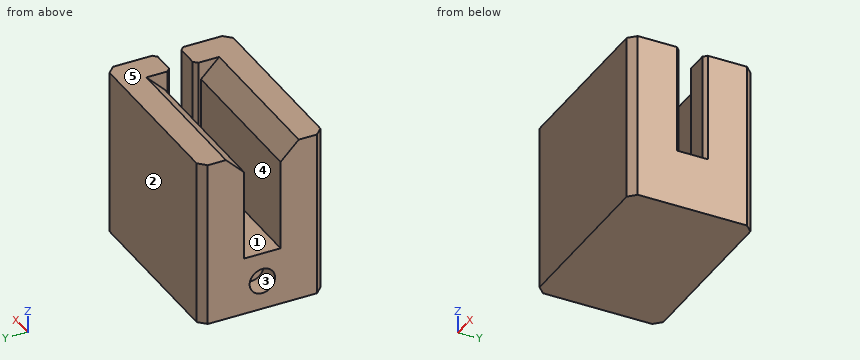
from build123d import *

# Parameters (mm, degrees)
F1_DEPTH = 34
F2_W     = 6.5
F2_H     = 30
F3_DEPTH = 8
F4_R     = 3.5
F5_DEPTH = 6
F6_W     = 42
F6_H     = 12
F7_DEPTH = 30
F8_SIZE  = 5
F9_SIZE  = 2
F10_SIZE = 1


with BuildPart() as f1:
    # F0 (on Front) → F1 (new body)
    with BuildSketch(Plane.XZ):
        Polygon((-20, 8), (-25, 8), (-25, -8), (25, -8), (25, 38), (17, 38), (17, 8), align=None)
    extrude(amount=F1_DEPTH)

    # F2 (on face) → F3 (cut, through all)
    with BuildSketch(Plane.YZ.offset(25)):
        with Locations((-17, 23)):
            Rectangle(F2_W, F2_H)
    extrude(amount=-F3_DEPTH, mode=Mode.SUBTRACT)

    # F4 (on face) → F5 (cut)
    with BuildSketch(Plane(origin=(-25, 0, 0), x_dir=(0, -1, 0), z_dir=(-1, 0, 0))):
        with Locations((17, 0)):
            Circle(F4_R)
    extrude(amount=-F5_DEPTH, mode=Mode.SUBTRACT)

    # F6 (on face) → F7 (join, through all)
    with BuildSketch(Plane.XY.offset(8)):
        with Locations((-4, -28)):
            Rectangle(F6_W, F6_H)
        with Locations((-4, -6)):
            Rectangle(F6_W, F6_H)
    extrude(amount=F7_DEPTH)

    # F8
    f8_edges = [f1.edges().sort_by_distance(p)[0] for p in [
        (-4, -22, 38),
        (-4, -12, 38),
    ]]
    chamfer(f8_edges, length=F8_SIZE)

    # F9
    f9_edges = [f1.edges().sort_by_distance(p)[0] for p in [
        (25, -34, 15),
        (25, 0, 15),
        (-25, -34, 15),
        (-25, 0, 15),
    ]]
    chamfer(f9_edges, length=F9_SIZE)

    # F10
    f10_edges = [f1.edges().sort_by_distance(p)[0] for p in [
        (17, -13.75, 23),
        (17, -20.25, 23),
        (25, -13.75, 23),
        (25, -20.25, 23),
    ]]
    chamfer(f10_edges, length=F10_SIZE)


solid = f1.part
Source: CAD feature listing. Evaluate the final solid. Frame: model axes, mm. Face numbers are marked on the shaded views. A direction names the side the tool comes from. Give positions to 0.01 mm unless a question says otherwise; leave off trailing zeros. Loops run counter-clockwise (first coordinate to the right, second up) from the corner with the lowest first, then second, coordinate; pieces in that order, holes last. Notation, with made-up numbers: (39, 12.5) -> (50, 12.5) arc R11 ccw to (50, 26.5) -> close; hole circle Ø8 at (75.25, -40). An arc over 180 degrees is marked (long way). Use a Markdown table: item, result. Add a question column.
1) Section query C-C, the plane z = 35. Return the cut outline in (x, y).
2) First-contact query: pin 1 (4 mm diameter, centred on x = -20, y = -11, fed in from +Z); pin 2 (1 mm diameter, centred on x = 16, y = -20, fed in from +Z); pin 3 (2 mm diameter, centred on y = -18, z = -1, fed in from -X); pin 4 (11 mm diameter, centred on y = -17, z = 0, fed in from -X). Flat tips, straight axial feed; report the tip coordinate or a pass-through.
3) Section query B-B, the plane x = -11. Return the cut outline in (y, z), then the cut area to 3 significant figures.
4) Section query D-D, the plane y = -17. Return the cut outline in (x, z).
5) Reachability of the marked faces 4 and 5 from +Z, -Z, +X, -X, +Y, -Y: full face, straight path, thin tool, end or side. Return the list, or none.
6) Section query A-A, the plane z = 27. Return the cut outline in (x, y).
7) Pull-direction query (Z, two-part tool) for the marked faces 1, 2 and 3; classes: +Z half, -Z half, draft (parallel to the pull), parting line (faces both ways), or undercut.
8) Line query: line 1 along Y through (x, z) = (14, 13.5); line 2 along Z through (x, y) = (-20.7, -17); line 3 along Z through (x, y) = (-11, -18). Output: solid intervals per line, ascending. Write a range as [from, to].
Numbers:
| question | item | result |
|---|---|---|
| 1 | outline | (-25, -32) -> (-23, -34) -> (23, -34) -> (25, -32) -> (25, -21.25) -> (24, -20.25) -> (18, -20.25) -> (17, -21.25) -> (17, -24) -> (-25, -24) -> close; (-25, -10) -> (17, -10) -> (17, -12.75) -> (18, -13.75) -> (24, -13.75) -> (25, -12.75) -> (25, -2) -> (23, 0) -> (-23, 0) -> (-25, -2) -> close |
| 2 | pin 1 | stops at z = 36 |
| 2 | pin 2 | stops at z = 8 |
| 2 | pin 3 | stops at x = -19 |
| 2 | pin 4 | stops at x = -25 |
| 3 | outline | (-34, -8) -> (0, -8) -> (0, 38) -> (-7, 38) -> (-12, 33) -> (-12, 8) -> (-22, 8) -> (-22, 33) -> (-27, 38) -> (-34, 38) -> close |
| 3 | area | 1,240 mm2 |
| 4 | outline | (-25, -8) -> (25, -8) -> (25, 8) -> (-25, 8) -> (-25, 3.5) -> (-19, 3.5) -> (-19, -3.5) -> (-25, -3.5) -> close |
| 5 | face 4 | +Z, -X |
| 5 | face 5 | +Z, +X, -X, +Y, -Y |
| 6 | outline | (-25, -32) -> (-23, -34) -> (23, -34) -> (25, -32) -> (25, -21.25) -> (24, -20.25) -> (18, -20.25) -> (17, -21.25) -> (17, -22) -> (-25, -22) -> close; (-25, -12) -> (17, -12) -> (17, -12.75) -> (18, -13.75) -> (24, -13.75) -> (25, -12.75) -> (25, -2) -> (23, 0) -> (-23, 0) -> (-25, -2) -> close |
| 7 | face 1 | +Z half |
| 7 | face 2 | draft |
| 7 | face 3 | undercut |
| 8 | line 1 | y = [-34, -22], [-12, 0] |
| 8 | line 2 | z = [-8, -3.5], [3.5, 8] |
| 8 | line 3 | z = [-8, 8] |
